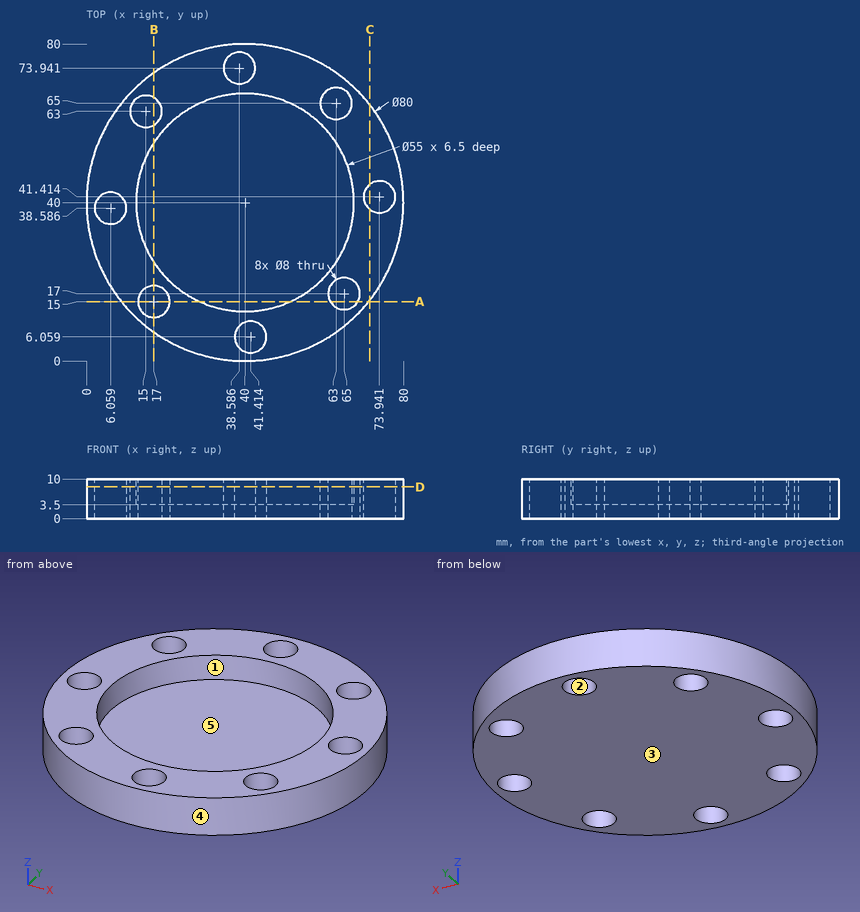
Geometry check sheet. Reference: drawing and pictorial views, mm from the part's lowest x, y, z. A direction names the side the tool comes from. Give positions to 0.01 mm unless a question says otherwise; leave off trailing zeros. Order: outer loops, then holes, each group sorted by start corner. A loop starts at its lowest first (then second) coordinate and runs counter-clockwise, first axis right, second up. Notation, with made-up numbers: M 32,-3.5 L 76,-3.5 A23 cw 76,6.5 Z; hole C 17.5,52 d2. An arc over 180 degrees is marked long. Use one line per item in the form item = value. Start each with the question number.
Q1. Mould release check, pull along X, two halves, no side actions. Record for the marked faces 3, 4 and 5: +X half, -X half, draft (parallel to the pull), parting line (faces both ways), or undercut.
Q2. Section check B-B (x = 17). Enter the section's corners in (y, z) (1 decimal), then the cut area to 3 significant figures.
Q3. Access from +Z, -Z, +X, -X, +Y, -Y to the whole of each face (thin tool, end or side, straight path). Record for the marked faces 1 and 2.
Q4. Section check C-C (x = 71.5). Enter the section's corners in (y, z), then the cut area to 3 significant figures.
Q5. Go/stop test with flat-tipped pins: pin 1 Ø5 at (x, y) = (73.94, 41.41) entering from -Z; pin 2 Ø2 at (x, y) = (46.5, 28) entering from +Z; pin 3 Ø5 at (y, z) = (22, 2.5) entering from -X (1 decimal). Record where each tip stops, or that it passes through.
Q6. Section check A-A (y = 15). Enter the section's corners in (x, z) (1 decimal), then the cut area to 3 significant figures.
Q7. Scan lines: line 1 along X through (y, z) = (17.5, 2.25); line 2 along Y through (x, z) = (37, 8). Record each from-to range of solid material in increasing order. Write a range as [from, to].
Q8. Section check D-D (z = 8). Count the separate pieces of the cut face and the enclosed holes in it, then the cut area to 3 significant figures.
Evaluation:
q1.face_3 = draft
q1.face_4 = parting line
q1.face_5 = undercut
q2.outline = M 7.3,0 L 11,0 L 11,10 L 7.3,10 Z; M 19,0 L 59.5,0 L 59.5,10 L 55.1,10 L 55.1,3.5 L 24.9,3.5 L 24.9,10 L 19,10 Z; M 66.5,0 L 72.7,0 L 72.7,10 L 66.5,10 Z
q2.area = 309 mm2
q3.face_1 = +Z
q3.face_2 = +Z, -Z
q4.outline = M 15.35,0 L 38.25,0 L 38.25,10 L 15.35,10 Z; M 44.58,0 L 64.65,0 L 64.65,10 L 44.58,10 Z
q4.area = 430 mm2
q5.pin_1 = through
q5.pin_2 = 3.5
q5.pin_3 = 3.1
q6.outline = M 8.8,0 L 13,0 L 13,10 L 8.8,10 Z; M 21,0 L 61.5,0 L 61.5,10 L 51.5,10 L 51.5,3.5 L 28.5,3.5 L 28.5,10 L 21,10 Z; M 68.5,0 L 71.2,0 L 71.2,10 L 68.5,10 Z
q6.area = 326 mm2
q7.line_1 = [6.93, 13.88], [20.12, 61.03], [68.97, 73.07]
q7.line_2 = [0.11, 12.66], [67.34, 70.27], [77.61, 79.89]
q8.separate_pieces = 1
q8.enclosed_holes = 9
q8.area = 2,250 mm2
